Solid Edge part; units mm, degrees
sketch "Sketch1" plane through (0, 0, 0) normal (0, 0, 1) x (1, 0, 0)
  line L0 (-5.4, -6.5) -> (5.4, -6.5)
  line L1 (5.4, -6.5) -> (5.4, 6.5)
  line L2 (5.4, 6.5) -> (-5.4, 6.5)
  line L3 (-5.4, 6.5) -> (-5.4, -6.5)
  dimension "D1" = 5.4
  dimension "D2" = 5.4
extrude "Protrusion1" add sketch "Sketch1" along normal blind 1.6
sketch "Sketch2" plane through (0, 0, 1.6) normal (0, 0, 1) x (1, 0, 0)
  circle A0 centre (3.05, 4.05) radius 1.45
extrude "Cutout1" cut sketch "Sketch2" against normal through all
sketch "Sketch3" plane through (0, 0, 1.6) normal (0, 0, 1) x (1, 0, 0)
  circle A0 centre (-3.75, -5.55) radius 0.45
  circle A1 centre (-1.25, -5.55) radius 0.45
  circle A2 centre (1.25, -5.55) radius 0.45
  circle A3 centre (3.75, -5.55) radius 0.45
extrude "Cutout2" cut sketch "Sketch3" against normal through all
sketch "Sketch4" plane through (0, 0, 0) normal (0, 0, -1) x (-1, 0, 0)
  line L0 (-0.1, 6.5) -> (-0.1, 0)
  line L1 (-0.1, 0) -> (-5.4, 0)
  line L2 (-5.4, 0) -> (-5.4, -3.7)
  line L3 (-5.4, -3.7) -> (5.4, -3.7)
  line L4 (5.4, -3.7) -> (5.4, 6.5)
  line L5 (5.4, 6.5) -> (-0.1, 6.5)
  dimension "D1" = 5.4
  dimension "D2" = 0.1
extrude "Extrusionsausprägung_2" add sketch "Sketch4" along normal blind 1
The listing builds one solid part. Answer for the finished solid, in the listing's coordinates (mm). A direction names the side the tool comes from. Coordinates: 2 decimals unless noted, no trailing zeros. Loops run counter-clockwise (first coordinate to the right, second up) from the corner with the lowest first, then second, coordinate; pieces in that order, holes last. Notation, with made-up numbers: (31, 43.5) -> (42, 43.5) arc R24 ccw to (42, 61.5) -> close; hole circle Ø1 at (23.25, -11). An arc over 180 degrees is marked (long way). Write item = value, one per line. Start each with the question number.
1) A cutting plane is placed at C-C (z = 1.4). Give the vertices of the cut face in (x, y).
2) A tool of negligible diameter and unlimited length cuts with its end or side. For faces 1 (the face through (2.7, 0, -0.5)), 2 (the face through (0.1, -3.7, -0.5)), 3 (the face through (0, -6.5, 1)), from which of +Z, -Z, +X, -X, +Y, -Y can it reach the whole face along a straight path? Write none if from no direction.
3) A cutting plane is placed at A-A (x = -1.25). Give the vertices of the cut face in (y, z).
4) A cutting plane is placed at D-D (y = -5.55). Give the vertices of the cut face in (x, z), then the cut area to 3 significant figures.
5) The mould has two halves that part along X. Classify faces 4 (the face through (0, -5, 0)), 5 (the face through (2.861, 5.488, 0.811)), 6 (the face through (1.46, -5.95, 0.81)), 7 (the face through (0.1, 3.3, -0.5)): released by +X, released by -X, zero draft, split by the parting line, or undercut.
6) Straight lines are drawn through the part: line 1 (Y direction, x = 3.75, z = 1); line 2 (Y direction, x = 3.05, z = 0.6); line 3 (Y direction, x = 1.25, z = 1.1). For each, find the intervals that lie inside material, in ascending order. Write a range as from..to.
7) Given pin 1 Ø0.5 at (x, z) = (2.5, -0.5) entering from +Y; pin 2 Ø0.8 at (x, z) = (1.5, -0.5) entering from -Y; pin 3 Ø1.4 at (x, y) = (2.5, -4.5) entering from -Z, each flat-ended and moving along its own axis, determine where each tip first touches the part or whether it passes through.
8) A cutting plane is placed at B-B (y = 4.05). Give the vertices of the cut face in (x, z).
Responses:
q1.outline = (-5.4, -6.5) -> (5.4, -6.5) -> (5.4, 6.5) -> (-5.4, 6.5) -> close; hole circle Ø0.9 at (-3.75, -5.55); hole circle Ø0.9 at (-1.25, -5.55); hole circle Ø0.9 at (1.25, -5.55); hole circle Ø2.9 at (3.05, 4.05); hole circle Ø0.9 at (3.75, -5.55)
q2.face_1 = -Z, +X, +Y
q2.face_2 = -Z, +X, -X, -Y
q2.face_3 = +Z, -Z, +X, -X, -Y
q3.outline = (-6.5, 0) -> (-6, 0) -> (-6, 1.6) -> (-6.5, 1.6) -> close; (-5.1, 0) -> (-3.7, 0) -> (-3.7, -1) -> (6.5, -1) -> (6.5, 1.6) -> (-5.1, 1.6) -> close
q4.outline = (-5.4, 0) -> (-4.2, 0) -> (-4.2, 1.6) -> (-5.4, 1.6) -> close; (-3.3, 0) -> (-1.7, 0) -> (-1.7, 1.6) -> (-3.3, 1.6) -> close; (-0.8, 0) -> (0.8, 0) -> (0.8, 1.6) -> (-0.8, 1.6) -> close; (1.7, 0) -> (3.3, 0) -> (3.3, 1.6) -> (1.7, 1.6) -> close; (4.2, 0) -> (5.4, 0) -> (5.4, 1.6) -> (4.2, 1.6) -> close
q4.area = 11.5 mm²
q5.face_4 = zero draft
q5.face_5 = undercut
q5.face_6 = undercut
q5.face_7 = released by +X
q6.line_1 = -6.5..-6, -5.1..2.78, 5.32..6.5
q6.line_2 = -6.5..2.6, 5.5..6.5
q6.line_3 = -6.5..-6, -5.1..6.5
q7.pin_1 = 0
q7.pin_2 = -3.7
q7.pin_3 = 0
q8.outline = (-5.4, -1) -> (0.1, -1) -> (0.1, 0) -> (1.6, 0) -> (1.6, 1.6) -> (-5.4, 1.6) -> close; (4.5, 0) -> (5.4, 0) -> (5.4, 1.6) -> (4.5, 1.6) -> close
